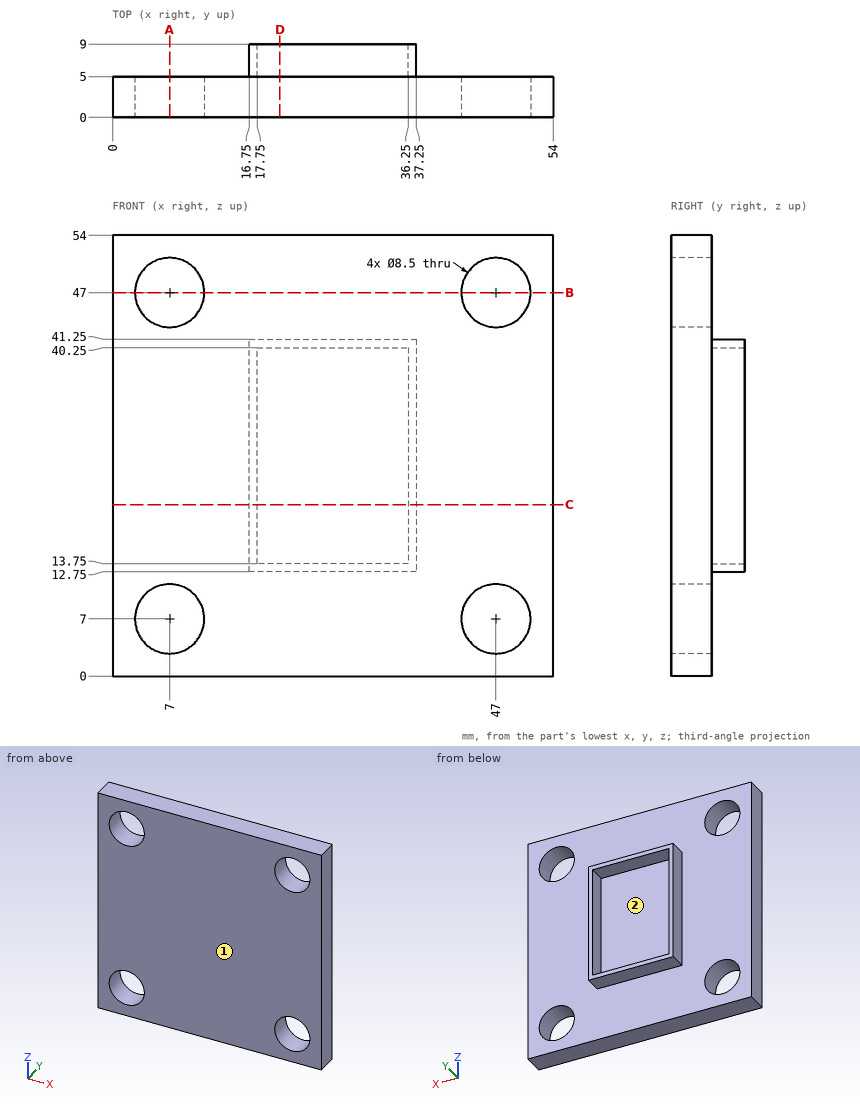
Part print with two shaded views. Sizes in mm from the minimum x, y, z corner. Round coordinates to 2 decimals unless told otherwise and drop trailing zeros. Order: outer loops, then holes, each group sorted by start corner. A loop starts at its lowest first (then second) coordinate and runs counter-clockwise, first axis right, second up. Notation, with made-up numbers: M -23.75,22 L 8.25,22 A24 cw 8.25,39 Z; hole C -19.5,-3 d3. An arc over 180 degrees is marked long. Use CSV: the item, a comma, the result in double quotes. Start each with the question number.
(1) Flat gauge pins, fed straight in: P1, Ø13.5, axis at x = 7, z = 7, coming from the +Y side; P2, Ø3, axis at x = 24, y = 7.5, coming from the -Z side; P3, Ø1.2, axis at x = 26.5, y = 6.5, coming from the +Z side. Where does each tip first touch, or does it go through?
(2) Mould opens along X. For the marked faces 1 and 2 say: +X half, -X half, draft (parallel to the pull), parting line (faces both ways), or undercut.
(3) Cut at C-C on z = 21. List the corners of the cut face in (x, y), then the cut area to 3 significant figures.
(4) Cut at B-B on z = 47. List the corners of the cut face in (x, y).
(5) Drill centre lines: probe 1 along X at (y, z) = (1.5, 47); probe 2 along Y at (x, z) = (10.5, 24). Where is each one in solid material? Low to high.
(6) Cut at D-D on x = 20.5. List the corners of the cut face in (y, z).
(7) Cut at A-A on x = 7. List the corners of the cut face in (y, z), then the cut area to 3 significant figures.
Findings:
1,P1,"stops at y = 5"
1,P2,"stops at z = 12.75"
1,P3,"stops at z = 41.25"
2,face 1,"draft"
2,face 2,"undercut"
3,outline,"M 0,0 L 54,0 L 54,5 L 37.25,5 L 37.25,9 L 36.25,9 L 36.25,5 L 17.75,5 L 17.75,9 L 16.75,9 L 16.75,5 L 0,5 Z"
3,area,"278 mm^2"
4,outline,"M 0,0 L 2.75,0 L 2.75,5 L 0,5 Z; M 11.25,0 L 42.75,0 L 42.75,5 L 11.25,5 Z; M 51.25,0 L 54,0 L 54,5 L 51.25,5 Z"
5,probe 1,"x = 0 to 2.75, 11.25 to 42.75, 51.25 to 54"
5,probe 2,"y = 0 to 5"
6,outline,"M 0,0 L 5,0 L 5,12.75 L 9,12.75 L 9,13.75 L 5,13.75 L 5,40.25 L 9,40.25 L 9,41.25 L 5,41.25 L 5,54 L 0,54 Z"
7,outline,"M 0,0 L 5,0 L 5,2.75 L 0,2.75 Z; M 0,11.25 L 5,11.25 L 5,42.75 L 0,42.75 Z; M 0,51.25 L 5,51.25 L 5,54 L 0,54 Z"
7,area,"185 mm^2"
